Work out the finished part from the listing and answer in its coordinate system (mm). Round coordinates to 2 decimals unless told otherwise and drop trailing zeros. Order: outer loops, then holes, each group sorted by start corner. A loop starts at its lowest first (then second) coordinate and runs counter-clockwise, first axis right, second up. Notation, with made-up numbers: (73, 55) - (94, 55) arc R33 ccw to (94, 91) - close; hole circle Ø11 at (20.25, 64.5). An arc over 180 degrees is marked (long way). Answer in a Markdown table with one row per item.
Autodesk Inventor part; units mm, degrees
ref_plane "YZ Plane" through (0, 0, 0) normal (1, 0, 0) x (0, 1, 0)
ref_plane "XZ Plane" through (0, 0, 0) normal (0, 1, 0) x (-1, 0, 0)
ref_plane "XY Plane" through (0, 0, 0) normal (0, 0, 1) x (1, 0, 0)
sketch "Sketch1" plane through (0, 0, 0) normal (0, 1, 0) x (-1, 0, 0)
  line L0 (0, 0) -> (38.1, 0)
  line L1 (38.1, 0) -> (38.1, 12.7)
  line L2 (38.1, 12.7) -> (0, 12.7)
  line L3 (0, 12.7) -> (0, 0)
  dimension "d0" = 38.1
  dimension "d1" = 12.7
extrude "Extrusion1" add sketch "Sketch1" along normal blind 38.1
sketch "Sketch2" plane through (0, 38.1, 0) normal (0, 1, 0) x (1, 0, 0)
  line L0 (0, 0) -> (-38.1, 0)
  line L1 (-38.1, -12.7) -> (0, -12.7)
  line L2 (-19.05, 0) -> (-19.05, -12.7) construction
  circle A0 centre (-31.75, -6.35) radius 3.7798
  circle A1 centre (-6.35, -6.35) radius 3.7798
  dimension "d4" = 12.7
hole "Hole1" at (-31.75, 38.1, 6.35) at (-6.35, 38.1, 6.35) direction (0, -1, 0) diameter 5.1054 end through all
sketch "Sketch3" plane through (-38.1, 0, 12.7) normal (0, 0, 1) x (1, 0, 0)
  line L0 (0, 38.1) -> (38.1, 38.1)
  circle A0 centre (19.05, 25.4) radius 3.652
  dimension "d12" = 12.7
hole "Hole2" at (-19.05, 25.4, 12.7) direction (0, 0, -1) diameter 5.1054 end through all
properties part number "hubjig_tab" material "Wood (Cherry)"
1) Find section A-A, the plane y = 25.4. Give the vertices of the cut face in (x, z), then the cut area to 3 significant figures.
Filled in:
| item | result |
|---|---|
| outline | (-38.1, 0) - (-21.6, 0) - (-21.6, 12.7) - (-38.1, 12.7) - close; (-16.5, 0) - (0, 0) - (0, 12.7) - (-16.5, 12.7) - close; hole circle Ø5.11 at (-31.75, 6.35); hole circle Ø5.11 at (-6.35, 6.35) |
| area | 378 mm^2 |
2) Find section D-D, the plane x = -19.05. Give the vertices of the cut face in (y, z).
Filled in:
| item | result |
|---|---|
| outline | (0, 0) - (22.85, 0) - (22.85, 12.7) - (0, 12.7) - close; (27.95, 0) - (38.1, 0) - (38.1, 12.7) - (27.95, 12.7) - close |
3) The mould has two halves that part along X. Classify faces 1 (the face through (-19, 0, 6)), 2 (the face through (-38.1, 19, 6)), 3 (the face through (-17.5, 27.43, 6.26)): released by +X, released by -X, zero draft, split by the parting line, or undercut.
Filled in:
| item | result |
|---|---|
| face 1 | zero draft |
| face 2 | released by -X |
| face 3 | undercut |
4) Find section C-C, the plane z = 4.5. Give the vertices of the cut face in (x, y), then the cut area to 3 significant figures.
Filled in:
| item | result |
|---|---|
| outline | (-38.1, 0) - (-33.51, 0) - (-33.51, 38.1) - (-38.1, 38.1) - close; (-29.99, 0) - (-8.11, 0) - (-8.11, 38.1) - (-29.99, 38.1) - close; (-4.59, 0) - (0, 0) - (0, 38.1) - (-4.59, 38.1) - close; hole circle Ø5.11 at (-19.05, 25.4) |
| area | 1,160 mm^2 |
5) This flat-tipped pin is pushed along its axis until it touches: pin 1 (4 mm diameter, centred on x = -6.35, z = 6.35, fed in from +Y). Where does it stop, or does it pass through?
Filled in:
| item | result |
|---|---|
| pin 1 | passes through |
6) Find the intervals of material crossed by probe 1 along X at (y, z) = (21, 6.35); probe 2 along Z at (x, y) = (-6.35, 27.5); probe 3 along X at (y, z) = (22, 5.75), in increasing order. Write a range as from..to.
Filled in:
| item | result |
|---|---|
| probe 1 | x = -38.1..-34.3, -29.2..-8.9, -3.8..0 |
| probe 2 | z = 0..3.8, 8.9..12.7 |
| probe 3 | x = -38.1..-34.23, -29.27..-8.83, -3.87..0 |
7) Find section B-B, the plane x = -31.75. Give the vertices of the cut face in (y, z), then the cut area to 3 significant figures.
Filled in:
| item | result |
|---|---|
| outline | (0, 0) - (38.1, 0) - (38.1, 3.8) - (0, 3.8) - close; (0, 8.9) - (38.1, 8.9) - (38.1, 12.7) - (0, 12.7) - close |
| area | 289 mm^2 |
